The listing builds one solid part. Answer for the finished solid, in the listing's coordinates (mm). Face numbers are marked on the shaded views. Give positions to 0.01 mm unless a question says otherwise; leave off trailing zeros. Order: outer loops, then holes, each group sorted by start corner. A loop starts at its lowest first (then second) coordinate and runs counter-clockwise, first axis right, second up. Notation, with made-up numbers: (33, 4) - (42, 4) arc R18 ccw to (42, 20) - close; hole circle Ø4 at (46.5, -1.75). An arc over 180 degrees is marked (long way). Answer in a Markdown table with one row per item.
from build123d import *

# Parameters (mm, degrees)
SKETCH1_W           = 18.84
SKETCH1_H           = 15
BOSS_EXTRUDE1_DEPTH = 3
CUT_EXTRUDE1_START  = -4
SKETCH2_R           = 2.4
CUT_EXTRUDE1_DEPTH  = 5


with BuildPart() as part:
    # Sketch1 → Boss-Extrude1 (new body)
    with BuildSketch(Plane(origin=(0, 0, 0), x_dir=(1, 0, 0), z_dir=(0, 1, 0))):
        Rectangle(SKETCH1_W, SKETCH1_H)
    extrude(amount=BOSS_EXTRUDE1_DEPTH)

    # Sketch2 → Cut-Extrude1 (cut)
    with BuildSketch(Plane(origin=(0, 3, 0), x_dir=(1, 0, 0), z_dir=(0, 1, 0)).offset(CUT_EXTRUDE1_START)):
        with Locations((-5, 0)):
            Circle(SKETCH2_R)
    cut_extrude1 = extrude(amount=CUT_EXTRUDE1_DEPTH, mode=Mode.SUBTRACT)

    # Mirror1: Cut-Extrude1 across plane
    add(cut_extrude1.mirror(Plane(origin=(0, 0, 0), x_dir=(0, 0, 1), z_dir=(1, 0, 0))), mode=Mode.SUBTRACT)


solid = part.part
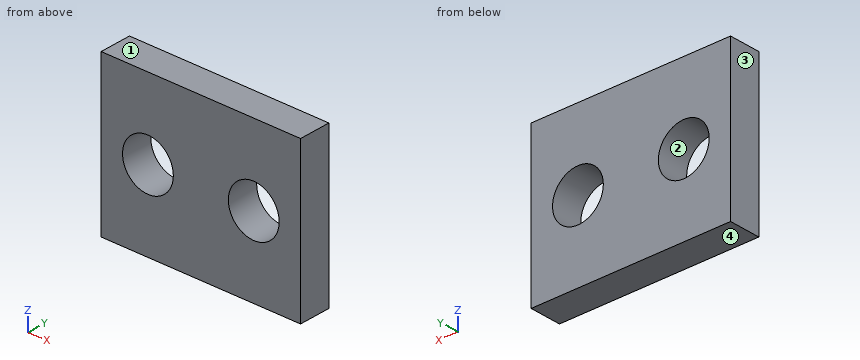
Item 1: Find section A-A on z = 0. Write down the section's boundary in (x, y), then the cut area to 3 significant figures.
Answer block:
| item | result |
|---|---|
| outline | (-9.42, 0) - (-7.4, 0) - (-7.4, 3) - (-9.42, 3) - close; (-2.6, 0) - (2.6, 0) - (2.6, 3) - (-2.6, 3) - close; (7.4, 0) - (9.42, 0) - (9.42, 3) - (7.4, 3) - close |
| area | 27.7 mm² |
Item 2: Consider line 1 (X direction, y = 0.25, z = 0.5); line 2 (Z direction, x = 5, y = 1.45); line 3 (X direction, y = 1.05, z = 1.5). Determine where each line is inside the solid, lowest interval first.
Answer block:
| item | result |
|---|---|
| line 1 | -9.42 to -7.35, -2.65 to 2.65, 7.35 to 9.42 |
| line 2 | -7.5 to -2.4, 2.4 to 7.5 |
| line 3 | -9.42 to -6.87, -3.13 to 3.13, 6.87 to 9.42 |
Item 3: Find section B-B on x = 5.75. Write down the section's boundary in (y, z), then the cut area to 3 significant figures.
Answer block:
| item | result |
|---|---|
| outline | (0, -7.5) - (3, -7.5) - (3, -2.28) - (0, -2.28) - close; (0, 2.28) - (3, 2.28) - (3, 7.5) - (0, 7.5) - close |
| area | 31.3 mm² |
Item 4: Determine the mould class of the marked faces 1, 2, 3 and 4 for opening direction Z: pulls with the +Z half, pulls with the -Z half, needs draft (parallel to the pull), parting line crosses it, or undercut.
Answer block:
| item | result |
|---|---|
| face 1 | pulls with the +Z half |
| face 2 | undercut |
| face 3 | needs draft |
| face 4 | pulls with the -Z half |
Item 5: Find section C-C on y = 2.05. Write down the section's boundary in (x, z), then the cut area to 3 significant figures.
Answer block:
| item | result |
|---|---|
| outline | (-9.42, -7.5) - (9.42, -7.5) - (9.42, 7.5) - (-9.42, 7.5) - close; hole circle Ø4.8 at (-5, 0); hole circle Ø4.8 at (5, 0) |
| area | 246 mm² |
